Design review of the part built by this model. Coordinates are the model's own, in mm. Round coordinates to 2 decimals unless told otherwise and drop trailing zeros. Order: outer loops, then holes, each group sorted by start corner. A loop starts at its lowest first (then second) coordinate and runs counter-clockwise, first axis right, second up.
from build123d import *

# Parameters (mm, degrees)
SKETCH1_W               = 130
SKETCH1_H               = 120
BOSS_EXTRUDE1_DEPTH     = 3
CUT_EXTRUDE1_START      = -4
SKETCH2_W               = 20
SKETCH2_H               = 95
CUT_EXTRUDE1_DEPTH      = 5
CUT_EXTRUDE2_START      = -4
SKETCH3_R               = 1.6
CUT_EXTRUDE2_DEPTH      = 5
SKETCH4_W               = 130
SKETCH4_H               = 3
BOSS_EXTRUDE2_DEPTH     = 140
SKETCH5_W               = 70
SKETCH5_H               = 6
CUT_EXTRUDE3_DEPTH      = 1
CUT_EXTRUDE3_DEPTH_BACK = 4
FILLET1_R               = 10


with BuildPart() as part:
    # Sketch1 → Boss-Extrude1 (new body)
    with BuildSketch(Plane(origin=(0, 0, 0), x_dir=(1, 0, 0), z_dir=(0, 1, 0))):
        Rectangle(SKETCH1_W, SKETCH1_H)
    extrude(amount=BOSS_EXTRUDE1_DEPTH)

    # Sketch2 → Cut-Extrude1 (cut)
    with BuildSketch(Plane(origin=(0, 3, 0), x_dir=(1, 0, 0), z_dir=(0, 1, 0)).offset(CUT_EXTRUDE1_START)):
        with Locations((-16.25, 0)):
            Rectangle(SKETCH2_W, SKETCH2_H)
    cut_extrude1 = extrude(amount=CUT_EXTRUDE1_DEPTH, mode=Mode.SUBTRACT)

    # Mirror1: Cut-Extrude1 across plane
    add(cut_extrude1.mirror(Plane(origin=(0, 0, 0), x_dir=(0, 0, 1), z_dir=(1, 0, 0))), mode=Mode.SUBTRACT)

    # Sketch3 → Cut-Extrude2 (cut)
    with BuildSketch(Plane(origin=(0, 3, 0), x_dir=(1, 0, 0), z_dir=(0, 1, 0)).offset(CUT_EXTRUDE2_START)):
        with Locations((44.5, 0)):
            Circle(SKETCH3_R)
    cut_extrude2 = extrude(amount=CUT_EXTRUDE2_DEPTH, mode=Mode.SUBTRACT)

    # Mirror2: Cut-Extrude2 across plane
    add(cut_extrude2.mirror(Plane(origin=(0, 0, 0), x_dir=(0, 0, 1), z_dir=(1, 0, 0))), mode=Mode.SUBTRACT)

    # Sketch4 → Boss-Extrude2 (add)
    with BuildSketch(Plane.XY.offset(60)):
        with Locations((0, 1.5)):
            Rectangle(SKETCH4_W, SKETCH4_H)
    extrude(amount=BOSS_EXTRUDE2_DEPTH)

    # Sketch5 → Cut-Extrude3 (cut, two sides)
    with BuildSketch(Plane(origin=(0, 3, 0), x_dir=(1, 0, 0), z_dir=(0, 1, 0))) as cut_extrude3_sk:
        with Locations((0, -75)):
            Rectangle(SKETCH5_W, SKETCH5_H)
        with Locations((0, -191)):
            Rectangle(SKETCH5_W, SKETCH5_H)
    extrude(amount=CUT_EXTRUDE3_DEPTH, mode=Mode.SUBTRACT)
    extrude(cut_extrude3_sk.sketch, amount=-CUT_EXTRUDE3_DEPTH_BACK, mode=Mode.SUBTRACT)

    # Fillet1
    fillet1_edges = [part.edges().sort_by_distance(p)[0] for p in [
        (-65, 1.5, 200),
        (65, 1.5, 200),
        (-65, 1.5, -60),
        (65, 1.5, -60),
    ]]
    fillet(fillet1_edges, radius=FILLET1_R)


solid = part.part
1) Clearance check with flat-ended pins moving along their axes: P1, Ø1, axis at x = 1.5, z = 26.5, coming from the -Y side; P2, Ø1.5, axis at y = 1.5, z = 192.5, coming from the -X side; P3, Ø1.5, axis at y = 1, z = 191.5, coming from the +X side. State where each tip first meets the part, or that it passes through.
Results:
P1: stops at y = 0
P2: stops at x = -64.85
P3: stops at x = 64.97
2) Take a section at A-A on z = -19.5. Give the boundary of the cut face in (x, y).
Results:
outline: (-65, 0) - (-26.25, 0) - (-26.25, 3) - (-65, 3) - close; (-6.25, 0) - (6.25, 0) - (6.25, 3) - (-6.25, 3) - close; (26.25, 0) - (65, 0) - (65, 3) - (26.25, 3) - close
3) Take a section at B-B on x = -19.5. Give the boundary of the cut face in (y, z).
Results:
outline: (0, -60) - (3, -60) - (3, -47.5) - (0, -47.5) - close; (0, 47.5) - (3, 47.5) - (3, 72) - (0, 72) - close; (0, 78) - (3, 78) - (3, 188) - (0, 188) - close; (0, 194) - (3, 194) - (3, 200) - (0, 200) - close
4) Take a section at D-D on y = 2.25. Give the boundary of the cut face in (x, z), plus the area to 3 significant figures.
Results:
outline: (-65, -50) arc R10 ccw to (-55, -60) - (55, -60) arc R10 ccw to (65, -50) - (65, 190) arc R10 ccw to (55, 200) - (-55, 200) arc R10 ccw to (-65, 190) - close; hole circle Ø3.2 at (-44.5, 0); hole (-35, 72) - (35, 72) - (35, 78) - (-35, 78) - close; hole (-35, 188) - (35, 188) - (35, 194) - (-35, 194) - close; hole (-26.25, -47.5) - (-6.25, -47.5) - (-6.25, 47.5) - (-26.25, 47.5) - close; hole (6.25, -47.5) - (26.25, -47.5) - (26.25, 47.5) - (6.25, 47.5) - close; hole circle Ø3.2 at (44.5, 0)
area: 29,100 mm2
5) Take a section at C-C on x = 0. Give the boundary of the cut face in (y, z), plus the area to 3 significant figures.
Results:
outline: (0, -60) - (3, -60) - (3, 72) - (0, 72) - close; (0, 78) - (3, 78) - (3, 188) - (0, 188) - close; (0, 194) - (3, 194) - (3, 200) - (0, 200) - close
area: 744 mm2
6) The part is to be moulded in two halves that separate along Z. For faces 1 (the face through (61.99, 1.52, 197.15)), 2 (the face through (-1, 3, 68)), 3 (the face through (61.99, 1.52, -57.15)), say which applies: released by +Z, released by -Z, zero draft, split by the parting line, or undercut.
Results:
face 1: released by +Z
face 2: zero draft
face 3: released by -Z
7) To check wall thickness, follow line 1 along Z through (x, y) = (29, 1.6); line 2 along X through (y, z) = (2.2, 25); line 3 along Z through (x, y) = (26, 1.8). State the ranges of each line that lie inside material, in increasing order.
Results:
line 1: z = -60 to 72, 78 to 188, 194 to 200
line 2: x = -65 to -26.25, -6.25 to 6.25, 26.25 to 65
line 3: z = -60 to -47.5, 47.5 to 72, 78 to 188, 194 to 200
